Check sheet for the modelled part. Datum: model origin and axes. Units: mm. A direction names the side the tool comes from. Give positions to 0.01 mm unless a question says otherwise; leave off trailing zeros. Order: outer loops, then holes, each group sorted by start corner. A loop starts at its lowest first (then second) coordinate and runs counter-clockwise, first axis right, second up. Notation, with made-up numbers: (46, 24) - (104, 24) arc R15 ccw to (104, 32) - close; hole circle Ø4 at (-10.5, -2.75). An arc over 180 degrees is marked (long way). Answer in a Markdown table with one row per item.
from build123d import *

# Parameters (mm, degrees)
SKETCH074_W  = 8.8
SKETCH074_H  = 11
SKETCH074_R  = 3.15
PAD098_DEPTH = 3.3
SKETCH072_R  = 3.15
PAD099_DEPTH = 9
PAD097_DEPTH = 1
SKETCH073_R  = 0.5
PAD096_DEPTH = 10


with BuildPart() as part:
    # Sketch074 → Pad098 (new body)
    with BuildSketch(Plane(origin=(0, -6.3, 0), x_dir=(-1, 0, 0), z_dir=(0, 1, 0))):
        with Locations((0, 5.5)):
            Rectangle(SKETCH074_W, SKETCH074_H)
        with Locations((0, 6.45)):
            Circle(SKETCH074_R, mode=Mode.SUBTRACT)
    extrude(amount=PAD098_DEPTH)

    # Sketch072 → Pad099 (join)
    with BuildSketch(Plane(origin=(0, -3, 0), x_dir=(-1, 0, 0), z_dir=(0, 1, 0))):
        with BuildLine():
            Line((4.4, 0), (-4.4, 0))
            Line((-4.4, 0), (-4.4, 6.45))
            ThreePointArc((4.4, 6.45), (0, 10.85), (-4.4, 6.45))
            Line((4.4, 6.45), (4.4, 0))
        make_face()
        with Locations((0, 6.45)):
            Circle(SKETCH072_R, mode=Mode.SUBTRACT)
    extrude(amount=PAD099_DEPTH)

    # Sketch075 → Pad097 (join)
    with BuildSketch(Plane(origin=(0, 6, 0), x_dir=(-1, 0, 0), z_dir=(0, 1, 0))):
        with BuildLine():
            Line((4.4, 0), (-4.4, 0))
            Line((-4.4, 0), (-4.4, 6.45))
            ThreePointArc((4.4, 6.45), (0, 10.85), (-4.4, 6.45))
            Line((4.4, 0), (4.4, 6.45))
        make_face()
    extrude(amount=PAD097_DEPTH)

    # Sketch073 → Pad096 (join)
    with BuildSketch(Plane(origin=(0, 6, 0), x_dir=(-1, 0, 0), z_dir=(0, 1, 0))):
        with Locations((0, 6.45)):
            Circle(SKETCH073_R)
    extrude(amount=-PAD096_DEPTH)


with BuildPart() as part_1:
    # Body015 placement: moved
    add(part.part.moved(Location((-2.8, -19.3, 0))))


solid = part_1.part
(1) Gauge pin test, flat ends, axial feed: P1, Ø1.1, axis at x = -3, z = 6.5, coming from the -Y side; P2, Ø4, axis at x = -5, y = -19, coming from the +Z side; P3, Ø2, axis at x = 0.5, y = -21, coming from the +Z side. Record the tip position at first contact, or that the pin passes through.
Geometry says:
| item | result |
|---|---|
| P1 | y = -23.3 |
| P2 | z = 10.85 |
| P3 | z = 10.2 |
(2) Cross-section at D-D, the plane z = 7.25. Record the cut outline in (x, y), then the cut area to 3 significant figures.
Geometry says:
| item | result |
|---|---|
| outline | (-7.2, -25.6) - (-5.85, -25.6) - (-5.85, -13.3) - (0.25, -13.3) - (0.25, -25.6) - (1.6, -25.6) - (1.6, -22.3) - (1.53, -22.3) - (1.53, -12.3) - (-7.13, -12.3) - (-7.13, -22.3) - (-7.2, -22.3) - close |
| area | 40.6 mm² |
(3) Cross-section at C-C, the plane y = -24. Record the cut outline in (x, z), then the cut area to 3 significant figures.
Geometry says:
| item | result |
|---|---|
| outline | (-7.2, 0) - (1.6, 0) - (1.6, 11) - (-7.2, 11) - close; hole circle Ø6.3 at (-2.8, 6.45) |
| area | 65.6 mm² |
(4) Mould release check, pull along X, two halves, no side actions. Record for faces 4 (the flat face through (-2, -13.3, 6)), 5 (the flat face through (-2.8, -23.3, 6.5)), 6 (the flat face through (-3, -19, 0)), 7 (the flat face through (1.6, -21, 4)): pulls with the +X half, pulls with the -X half, needs draft (parallel to the pull), parting line crosses it, or undercut.
Geometry says:
| item | result |
|---|---|
| face 4 | undercut |
| face 5 | undercut |
| face 6 | needs draft |
| face 7 | pulls with the +X half |
(5) Cross-section at B-B, the plane x = -2.8. Record the cut outline in (y, z), then the cut area to 3 significant figures.
Geometry says:
| item | result |
|---|---|
| outline | (-25.6, 0) - (-12.3, 0) - (-12.3, 10.85) - (-22.3, 10.85) - (-22.3, 11) - (-25.6, 11) - (-25.6, 9.6) - (-13.3, 9.6) - (-13.3, 6.95) - (-23.3, 6.95) - (-23.3, 5.95) - (-13.3, 5.95) - (-13.3, 3.3) - (-25.6, 3.3) - close |
| area | 77.3 mm² |
(6) Cross-section at A-A, the plane y = -16.5. Record the cut outline in (x, z).
Geometry says:
| item | result |
|---|---|
| outline | (-7.2, 0) - (1.6, 0) - (1.6, 6.45) arc R4.4 ccw to (-7.2, 6.45) - close; circle Ø1 at (-2.8, 6.45); hole circle Ø6.3 at (-2.8, 6.45) |
(7) Thickness scan on L1, parallel to Z at x = -2.8, y = -17.5; L2, parallel to X at y = -20.5, z = 6.5; L3, parallel to Z at x = -2.8, y = -22.5. Record the ranges inside material, lowest first.
Geometry says:
| item | result |
|---|---|
| L1 | 0 to 3.3, 5.95 to 6.95, 9.6 to 10.85 |
| L2 | -7.2 to -5.95, -3.3 to -2.3, 0.35 to 1.6 |
| L3 | 0 to 3.3, 5.95 to 6.95, 9.6 to 11 |
(8) Access from +Z, -Z, +X, -X, +Y, -Y to the whole of each face (thin tool, end or side, straight path). Record for faces 1 (the cylindrical face through (-2.735, -18.23, 6.946)), 2 (the cylindrical face through (-2.9, -17.37, 10.85)), 3 (the flat face through (-3, -24, 11)).
Geometry says:
| item | result |
|---|---|
| face 1 | -Y |
| face 2 | +Z, +Y |
| face 3 | +Z, +X, -X, +Y, -Y |
